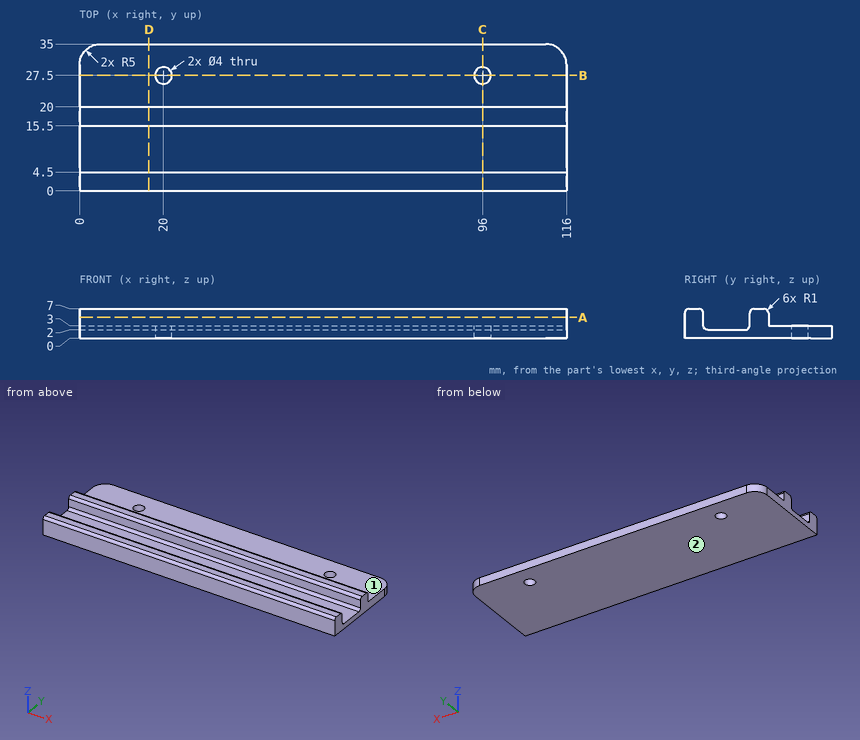
Print and shaded views of the part. All mm, measured from the part's lowest x, y and z. A direction names the side the tool comes from. Coordinates: 2 decimals unless noted, no trailing zeros. Loops run counter-clockwise (first coordinate to the right, second up) from the corner with the lowest first, then second, coordinate; pieces in that order, holes last. Notation, with made-up numbers: M 73,-1.75 L 106,-1.75 A33 cw 106,35.25 Z; hole C 44.5,72.25 d2. An arc over 180 degrees is marked long. Use a Markdown table: item, result. Add a question column.
Q1. Cut at C-C (x = 96). Write the cut outline in (y, z), and give its area (3 significant figures).
Q2. Cut at A-A (z = 5). Write the cut outline in (x, y), and give its area (3 significant figures).
Q3. Probe L1, parallel to Y at x = 44.5, z = 4.75; L2, parallel to X at y = 26.5, z = 2.75; L3, parallel to Z at x = 48, y = 27.5. List the from-to ranges inside material, lowest first.
Q4. Cut at B-B (y = 27.5). Write the cut outline in (x, z).
Q5. Which spindle directions (+Z, -Z, +X, -X, +Y, -Y) get a long thin tool onto all of the face, cutting with end or side? Do the marked faces 1 and 2. Say none if no direction does.
Q6. Pin check, flat tips, straight feed: P1, Ø3, axis at x = 96, y = 27.5, coming from the +Z side; P2, Ø4.5, axis at x = 55.5, y = 11, coming from the +Z side. Stop position of each tip, or through.
Q7. Cut at D-D (x = 16.5). Write the cut outline in (y, z).
Worked out:
| question | item | result |
|---|---|---|
| 1 | outline | M 0,0 L 25.5,0 L 25.5,3 L 20,3 L 20,6 A1 ccw 19,7 L 16.5,7 A1 ccw 15.5,6 L 15.5,3 A1 cw 14.5,2 L 5.5,2 A1 cw 4.5,3 L 4.5,6 A1 ccw 3.5,7 L 1,7 A1 ccw 0,6 Z; M 29.5,0 L 35,0 L 35,3 L 29.5,3 Z |
| 1 | area | 118 mm2 |
| 2 | outline | M 0,0 L 116,0 L 116,4.5 L 0,4.5 Z; M 0,15.5 L 116,15.5 L 116,20 L 0,20 Z |
| 2 | area | 1,040 mm2 |
| 3 | L1 | y = 0 to 4.5, 15.5 to 20 |
| 3 | L2 | x = 0 to 18.27, 21.73 to 94.27, 97.73 to 116 |
| 3 | L3 | z = 0 to 3 |
| 4 | outline | M 0,0 L 18,0 L 18,3 L 0,3 Z; M 22,0 L 94,0 L 94,3 L 22,3 Z; M 98,0 L 116,0 L 116,3 L 98,3 Z |
| 5 | face 1 | +Z, +X, -X, +Y |
| 5 | face 2 | -Z, +X, -X, +Y, -Y |
| 6 | P1 | passes through |
| 6 | P2 | stops at z = 2 |
| 7 | outline | M 0,0 L 35,0 L 35,3 L 20,3 L 20,6 A1 ccw 19,7 L 16.5,7 A1 ccw 15.5,6 L 15.5,3 A1 cw 14.5,2 L 5.5,2 A1 cw 4.5,3 L 4.5,6 A1 ccw 3.5,7 L 1,7 A1 ccw 0,6 Z |
